Build history of the part. All positions in model axes, mm. A direction names the side the tool comes from. Give positions to 0.01 mm unless a question says otherwise; leave off trailing zeros. Loops run counter-clockwise (first coordinate to the right, second up) from the corner with the lowest first, then second, coordinate; pieces in that order, holes last. Notation, with made-up numbers: M 26.5,18.25 L 32.5,18.25 A19 cw 32.5,53.25 Z; hole C 83.25,79.25 d9. An arc over 180 degrees is marked long. Put each result on its own line as item: value.
```python
from build123d import *

# Parameters (mm, degrees)
F1_DEPTH = 9.525
F2_R     = 5.08
F3_R     = 3.175
F4_DEPTH = 25.4
F5_R     = 3.175
F6_DEPTH = 7.62
F7_R     = 3.175
F8_DEPTH = 7.62


with BuildPart() as f1:
    # F0 (on Front) → F1 (new body, symmetric)
    with BuildSketch(Plane.XZ):
        Polygon((-19.05, 50.8), (-22.225, 0), (22.225, 0), (19.05, 50.8), align=None)
    extrude(amount=F1_DEPTH, both=True)

    # F2
    f2_edges = [f1.edges().sort_by_distance(p)[0] for p in [
        (0, -9.525, 50.8),
        (19.05, 0, 50.8),
        (-19.05, 0, 50.8),
        (0, 9.525, 50.8),
        (22.225, 0, 0),
        (0, -9.525, 0),
        (-22.225, 0, 0),
        (0, 9.525, 0),
        (20.6375, -9.525, 25.4),
        (20.6375, 9.525, 25.4),
        (-20.6375, 9.525, 25.4),
        (-20.6375, -9.525, 25.4),
    ]]
    fillet(f2_edges, radius=F2_R)

    # F3 (on Right) → F4 (cut, symmetric)
    with BuildSketch(Plane.YZ):
        with Locations((0, 39.686882)):
            Circle(F3_R)
    extrude(amount=F4_DEPTH, both=True, mode=Mode.SUBTRACT)

    # F5 (on face) → F6 (cut)
    with BuildSketch(Plane.XY.offset(50.8)):
        Circle(F5_R)
    extrude(amount=-F6_DEPTH, mode=Mode.SUBTRACT)

    # F7 (on face) → F8 (cut)
    with BuildSketch(Plane(origin=(0, 0, 0), x_dir=(1, 0, 0), z_dir=(0, 0, -1))):
        with Locations((-9.525, 0)):
            Circle(F7_R)
        with Locations((9.525, 0)):
            Circle(F7_R)
    extrude(amount=-F8_DEPTH, mode=Mode.SUBTRACT)


solid = f1.part
```
Q1. Slice it at B-B (z = 4). List the corners of the cut face in (x, y) (3 decimals), and give its area (3 significant figures).
Here are the results:
outline: M -21.781,-4.445 A4.964 ccw -16.818,-9.409 L 16.818,-9.409 A4.964 ccw 21.781,-4.445 L 21.781,4.445 A4.964 ccw 16.818,9.409 L -16.818,9.409 A4.964 ccw -21.781,4.445 Z; hole C -9.525,0 d6.35; hole C 9.525,0 d6.35
area: 735 mm²
Q2. Slice it at C-C (x = -2). List the corners of the cut face in (y, z) (3 decimals).
Here are the results:
outline: M -9.525,5.08 A5.08 ccw -4.445,0 L 4.445,0 A5.08 ccw 9.525,5.08 L 9.525,45.72 A5.08 ccw 4.445,50.8 L 2.466,50.8 L 2.466,43.18 L -2.466,43.18 L -2.466,50.8 L -4.445,50.8 A5.08 ccw -9.525,45.72 Z; hole C 0,39.687 d6.35
Q3. Drop flat-ended pins along their axis: pin 1 Ø7 at (x, y) = (-11, 1) entering from -Z; pin 2 Ø3 at (x, y) = (0.5, -0.5) entering from +Z; pin 3 Ø2 at (y, z) = (-5.5, 21) entering from +X; pin 4 Ø4 at (x, y) = (-9.525, 0) entering from -Z. Give the stop position or say it passes through.
Here are the results:
pin 1: z = 0
pin 2: z = 43.18
pin 3: x = 20.94
pin 4: z = 7.62
Q4. Probe line 1 (Y direction, x = 0, z = 45) (3 decimals); line 2 (Z direction, x = -10, y = 0); line 3 (X direction, y = 0, z = 1.5). List the from-to ranges inside material, lowest first. Write a range as from..to.
Here are the results:
line 1: -9.525..-3.175, 3.175..9.525
line 2: 7.62..36.51, 42.86..50.8
line 3: -20.42..-12.7, -6.35..6.35, 12.7..20.42
Q5. Slice it at D-D (y = 5.5). List the corners of the cut face in (x, z).
Here are the results:
outline: M -21.78,5.39 A4.97 ccw -16.82,0.11 L 16.82,0.11 A4.97 ccw 21.78,5.39 L 19.24,46.03 A4.97 ccw 14.28,50.69 L -14.28,50.69 A4.97 ccw -19.24,46.03 Z
Q6. Slice it at A-A (y = 0). List the corners of the cut face in (x, z) (3 decimals), and give its area (3 significant figures).
Here are the results:
outline: M -21.888,5.397 A5.08 ccw -16.818,0 L -12.7,0 L -12.7,7.62 L -6.35,7.62 L -6.35,0 L 6.35,0 L 6.35,7.62 L 12.7,7.62 L 12.7,0 L 16.818,0 A5.08 ccw 21.888,5.397 L 19.943,36.512 L -19.943,36.512 Z; M -19.546,42.862 L 19.546,42.862 L 19.348,46.037 A5.08 ccw 14.278,50.8 L 3.175,50.8 L 3.175,43.18 L -3.175,43.18 L -3.175,50.8 L -14.278,50.8 A5.08 ccw -19.348,46.037 Z
area: 1,680 mm²
Q7. Tool access for faces 5 (the cylindrical face through (-0.69, -3.1, 47.04)), 6 (the cylindrical face through (19.15, 8, 25.91)), 7 (the flat face through (-10, 0, 7.62)): list every direction of +Z, -Z, +X, -X, +Y, -Y with a clear straight run to the whole face (end or side of a thin tool).
Here are the results:
face 5: +Z
face 6: +Z, +X, +Y
face 7: -Z
Q8. Mould opens along Y. For faces 1 (the flat face through (9, 0, 7.62)), 2 (the cylindrical face through (-17.79, 0.06, 49.39)), 3 (the cylindrical face through (-12.045, 1.932, 3.757)), 4 (the cylindrical face through (19.15, -8, 25.91)) say: pulls with the +Y half, pulls with the -Y half, needs draft (parallel to the pull), parting line crosses it, or undercut.
Here are the results:
face 1: undercut
face 2: needs draft
face 3: undercut
face 4: pulls with the -Y half
